Could you check a few things on this model? Use its own coordinates, in mm. Coordinates: 2 decimals unless noted, no trailing zeros. Write each loop counter-clockwise with the first axis right and the second up, starting at its lowest first coordinate (ties: lowest second). Pieces come first, ordered by that corner, then holes.
```python
from build123d import *

# Parameters (mm, degrees)
SKETCH_1_W          = 450
SKETCH_1_H          = 25
EXTRUDE_1_DEPTH     = 3
SKETCH_2_W          = 53
SKETCH_2_H          = 30
SKETCH_2_R          = 2
EXTRUDE_2_DEPTH     = 3
SKETCH_3_R          = 5.655027455
CUT_EXTRUDE_1_DEPTH = 454.358577728


with BuildPart() as part:
    # 草图1 → 凸台-拉伸1 (new body)
    with BuildSketch(Plane(origin=(0, 0, 0), x_dir=(0, 0, -1), z_dir=(1, 0, 0))):
        with Locations((225, 12.5)):
            Rectangle(SKETCH_1_W, SKETCH_1_H)
    extrude(amount=EXTRUDE_1_DEPTH)

    # 草图2 → 凸台-拉伸2 (add)
    # profile 1 of 2: a face of its own
    with BuildSketch(Plane(origin=(3, 0, 0), x_dir=(0, 0, -1), z_dir=(1, 0, 0))):
        with Locations((82, 40)):
            Rectangle(SKETCH_2_W, SKETCH_2_H)
        with Locations((58.5, 44.5)):
            Circle(SKETCH_2_R, mode=Mode.SUBTRACT)
        with Locations(Location((105.5, 44.5, 0), (0, 0, 180))):
            Circle(SKETCH_2_R, mode=Mode.SUBTRACT)
    # profile 2 of 2: a face of its own
    with BuildSketch(Plane(origin=(3, 0, 0), x_dir=(0, 0, -1), z_dir=(1, 0, 0))):
        with Locations((368, 40)):
            Rectangle(SKETCH_2_W, SKETCH_2_H)
        with Locations((344.5, 44.5)):
            Circle(SKETCH_2_R, mode=Mode.SUBTRACT)
        with Locations(Location((391.5, 44.5, 0), (0, 0, 180))):
            Circle(SKETCH_2_R, mode=Mode.SUBTRACT)
    extrude(amount=-EXTRUDE_2_DEPTH)

    # 草图3 → 切除-拉伸1 (cut, through all)
    with BuildSketch(Plane(origin=(3, 0, 0), x_dir=(0, 0, -1), z_dir=(1, 0, 0))):
        with Locations((225, 12.5)):
            Circle(SKETCH_3_R)
        with Locations((315, 12.5)):
            Circle(SKETCH_3_R)
        with Locations((405, 12.5)):
            Circle(SKETCH_3_R)
        with Locations((135, 12.5)):
            Circle(SKETCH_3_R)
        with Locations((45, 12.5)):
            Circle(SKETCH_3_R)
    extrude(amount=-CUT_EXTRUDE_1_DEPTH, mode=Mode.SUBTRACT)


solid = part.part
```
1. Please list where these lines run through material, in increasing order: line 1 along Z through (x, y) = (1.3, 44); line 2 along Z through (x, y) = (0.8, 47); line 3 along Y through (x, z) = (1.05, -58.5).
Verdict:
line 1: z = -394.5 to -393.44, -389.56 to -346.44, -342.56 to -341.5, -108.5 to -107.44, -103.56 to -60.44, -56.56 to -55.5
line 2: z = -394.5 to -341.5, -108.5 to -55.5
line 3: y = 0 to 42.5, 46.5 to 55
2. For pin 1 (5 mm diameter, centred on y = 44.5, z = -344.5, fed in from +X); pin 2 (0.9 mm diameter, centred on x = 1, z = -26.5, fed in from +Y), each with a flat end and sliding along its axis, tell me the tip position at first contact or that it passes through.
Verdict:
pin 1: stops at x = 3
pin 2: stops at y = 25
3. I want a section at D-D on y = 37.5. Please give me the cut outline in (x, z), plus the area to 3 significant figures.
Verdict:
outline: (0, -394.5) - (3, -394.5) - (3, -341.5) - (0, -341.5) - close; (0, -108.5) - (3, -108.5) - (3, -55.5) - (0, -55.5) - close
area: 318 mm2
4. I want a section at A-A on z = -225. Please give me the cut outline in (x, y), plus the area to 3 significant figures.
Verdict:
outline: (0, 0) - (3, 0) - (3, 6.84) - (0, 6.84) - close; (0, 18.16) - (3, 18.16) - (3, 25) - (0, 25) - close
area: 41.1 mm2
5. I want a section at B-B on x = 2.45. Give the number of separate pieces and of enclosed holes in the cut face, plus the area to 3 significant figures.
Verdict:
separate pieces: 1
enclosed holes: 9
area: 13,900 mm2
6. If we mould it in two halves opening along Y, with no side actions, what happens to faces 1 (the face through (1.521, 14.199, -140.394)), 2 (the face through (0, 22, -222))? For each: pulls with the +Y half, pulls with the -Y half, needs draft (parallel to the pull), parting line crosses it, or undercut.
Verdict:
face 1: undercut
face 2: needs draft
7. I want a section at C-C on y = 12.5. Please give me the cut outline in (x, z), plus the area to 3 significant figures.
Verdict:
outline: (0, -450) - (3, -450) - (3, -410.66) - (0, -410.66) - close; (0, -399.34) - (3, -399.34) - (3, -320.66) - (0, -320.66) - close; (0, -309.34) - (3, -309.34) - (3, -230.66) - (0, -230.66) - close; (0, -219.34) - (3, -219.34) - (3, -140.66) - (0, -140.66) - close; (0, -129.34) - (3, -129.34) - (3, -50.66) - (0, -50.66) - close; (0, -39.34) - (3, -39.34) - (3, 0) - (0, 0) - close
area: 1,180 mm2
